```python
from build123d import *

# Parameters (mm, degrees)
SKETCH_1_R          = 11.5
EXTRUDE_1_DEPTH     = 10
SKETCH_2_R          = 10
SKETCH_2_R_2        = 3.5
CUT_EXTRUDE_1_DEPTH = 9
SKETCH_3_R          = 2.5
CUT_EXTRUDE_2_DEPTH = 1
CUT_EXTRUDE_START   = -1
SKETCH_4_R          = 2.5
CUT_EXTRUDE_3_DEPTH = 1
SKETCH_5_R          = 2
CUT_EXTRUDE_4_DEPTH = 19.587630295
CHAMFER_1_SIZE      = 1
CHAMFER_2_SIZE      = 0.5


with BuildPart() as part:
    # 草图1 → 凸台-拉伸1 (new body)
    with BuildSketch(Plane(origin=(0, 0, 0), x_dir=(1, 0, 0), z_dir=(0, 1, 0))):
        with Locations(Location((0, 0, 0), (0, 0, 270))):
            Circle(SKETCH_1_R)
    extrude(amount=EXTRUDE_1_DEPTH)

    # 草图2 → 切除-拉伸1 (cut)
    with BuildSketch(Plane(origin=(0, 10, 0), x_dir=(1, 0, 0), z_dir=(0, 1, 0))):
        with Locations(Location((0, 0, 0), (0, 0, 270))):
            Circle(SKETCH_2_R)
        with Locations(Location((0, 0, 0), (0, 0, 270))):
            Circle(SKETCH_2_R_2, mode=Mode.SUBTRACT)
    extrude(amount=-CUT_EXTRUDE_1_DEPTH, mode=Mode.SUBTRACT)

    # 草图3 → 切除-拉伸2 (cut)
    with BuildSketch(Plane(origin=(0, 10, 0), x_dir=(1, 0, 0), z_dir=(0, 1, 0))):
        with Locations(Location((0, 0, 0), (0, 0, 270))):
            Circle(SKETCH_3_R)
    extrude(amount=-CUT_EXTRUDE_2_DEPTH, mode=Mode.SUBTRACT)

    # 草图4 → 切除-拉伸3 (cut)
    with BuildSketch(Plane.XZ.offset(CUT_EXTRUDE_START)):
        with Locations(Location((0, 0, 0), (0, 0, 90))):
            Circle(SKETCH_4_R)
    extrude(amount=CUT_EXTRUDE_3_DEPTH, mode=Mode.SUBTRACT)

    # 草图5 → 切除-拉伸4 (cut, through all)
    with BuildSketch(Plane.XZ.offset(-1)):
        with Locations(Location((0, 0, 0), (0, 0, 270))):
            Circle(SKETCH_5_R)
    extrude(amount=-CUT_EXTRUDE_4_DEPTH, mode=Mode.SUBTRACT)

    # 倒角1
    chamfer_1_edges = [part.edges().sort_by_distance(p)[0] for p in [
        (0, 0, -11.5),
        (0, 10, -11.5),
    ]]
    chamfer(chamfer_1_edges, length=CHAMFER_1_SIZE)

    # 倒角2
    chamfer_2_edges = [part.edges().sort_by_distance(p)[0] for p in [
        (0, 10, -3.5),
    ]]
    chamfer(chamfer_2_edges, length=CHAMFER_2_SIZE)


solid = part.part
```
Part model, mm, in its own coordinate system. A direction names the side the tool comes from. Round coordinates to 2 decimals unless told otherwise and drop trailing zeros. Loops run counter-clockwise (first coordinate to the right, second up) from the corner with the lowest first, then second, coordinate; pieces in that order, holes last. Notation, with made-up numbers: (-15, -29.5) -> (27, -29.5) arc R16 cw to (27, -15.5) -> close; hole circle Ø9 at (73, 59). An arc over 180 degrees is marked (long way). Use CSV: the item, a comma, the result in double quotes. Start each with the question number.
1) Wall check: L1, parallel to X at y = 6, z = 0; L2, parallel to X at y = 9.6, z = 0; L3, parallel to Y at x = 6.5, z = -6.75. Give the ranges that are in metal, low to high. Write a range as [from, to].
2) Drop flat-ended pins along their axis: P1, Ø3, axis at x = 0, z = 0, coming from the -Y side; P2, Ø5, axis at x = 2.5, y = 4.5, coming from the -Z side; P3, Ø2.5, axis at x = 1, z = 0.5, coming from the +Y side; P4, Ø1.5, axis at y = 4, z = 6, coming from the -X side. Give the stop position or say it passes through.
3) Cut at C-C, the plane y = 3. Write the cut outline in (x, z), plus the area to 3 significant figures.
4) Pull direction Z, two halves, no side cores. Call faces 1 (the cylindrical face through (9.7, 4.94, 6.18)), 2 (the cylindrical face through (2.44, 0.51, -0.54)), 3 (the flat face through (2, 10, -2)): +Z half, -Z half, draft (parallel to the pull), parting line (faces both ways), or undercut.
5) Which spindle directions (+Z, -Z, +X, -X, +Y, -Y) get a long thin tool onto all of the face, cutting with end or side? Do faces 4 (the cylindrical face through (-2, 5, 0)), 5 (the flat face through (-2, 1, -1)), 6 (the cylindrical face through (-9.76, 5.56, -2.17)). Say none if no direction does.
Determined:
1,L1,"x = [-11.5, -10], [-3.5, -2], [2, 3.5], [10, 11.5]"
1,L2,"x = [-10.9, -10], [-3.4, -2.5], [2.5, 3.4], [10, 10.9]"
1,L3,"y = [0, 1]"
2,P1,"passes through"
2,P2,"stops at z = -11.5"
2,P3,"stops at y = 9"
2,P4,"stops at x = -10.23"
3,outline,"circle Ø23 at (0, 0); circle Ø7 at (0, 0); hole circle Ø20 at (0, 0); hole circle Ø4 at (0, 0)"
3,area,"127 mm2"
4,face 1,"parting line"
4,face 2,"undercut"
4,face 3,"draft"
5,face 4,"+Y, -Y"
5,face 5,"-Y"
5,face 6,"+Y"
